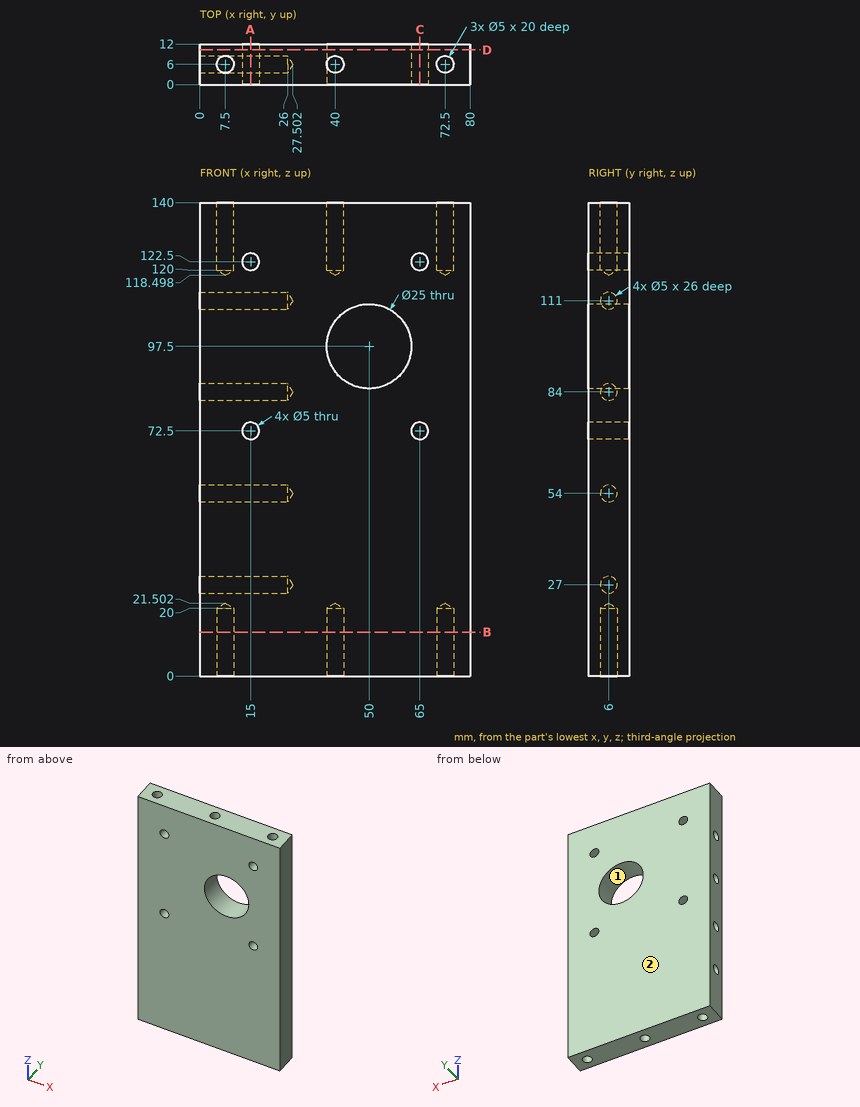
Here's the drawing with two shaded views (mm, measured from the low corner). I have some questions. Give positions to 0.01 mm unless a question says otherwise; leave off trailing zeros. Loops run counter-clockwise (first coordinate to the right, second up) from the corner with the lowest first, then second, coordinate; pieces in that order, holes last. Notation, with made-up numbers: (4, 20) - (52, 20) arc R35 cw to (52, 53) - close; hole circle Ø8 at (82, 28.5). An arc over 180 degrees is marked (long way). Return JSON: item names as keys, results as strings.
1. If I drill on line 1 (Z direction, x = 15, y = 3.25); line 2 (X direction, y = 6, z = 127); line 3 (Z direction, x = 18.75, y = 6), over which ranges is the centre line in solid material (lowest first)?
Output values:
{"line 1": "z = 0 to 70, 75 to 120, 125 to 140", "line 2": "x = 0 to 5, 10 to 37.5, 42.5 to 70, 75 to 80", "line 3": "z = 0 to 24.5, 29.5 to 51.5, 56.5 to 81.5, 86.5 to 108.5, 113.5 to 140"}
2. I want a section at D-D on y = 10.25. Please give me the cut outline in (x, z).
Output values:
{"outline": "(0, 0) - (80, 0) - (80, 140) - (0, 140) - close; hole circle Ø5 at (15, 72.5); hole circle Ø5 at (15, 122.5); hole circle Ø25 at (50, 97.5); hole circle Ø5 at (65, 72.5); hole circle Ø5 at (65, 122.5)"}
3. I want a section at C-C on x = 65. Please give me the cut outline in (y, z).
Output values:
{"outline": "(0, 0) - (12, 0) - (12, 70) - (0, 70) - close; (0, 75) - (12, 75) - (12, 120) - (0, 120) - close; (0, 125) - (12, 125) - (12, 140) - (0, 140) - close"}
4. I want a section at A-A on x = 15. Please give me the cut outline in (y, z).
Output values:
{"outline": "(0, 0) - (12, 0) - (12, 70) - (0, 70) - close; (0, 75) - (12, 75) - (12, 120) - (0, 120) - close; (0, 125) - (12, 125) - (12, 140) - (0, 140) - close; hole circle Ø5 at (6, 27); hole circle Ø5 at (6, 54); hole circle Ø5 at (6, 84); hole circle Ø5 at (6, 111)"}
5. We'd pull the mould along X, two halves only. Please class the marked faces 1 and 2: +X half, -X half, draft (parallel to the pull), parting line (faces both ways), or undercut.
Output values:
{"face 1": "undercut", "face 2": "draft"}
6. I want a section at B-B on z = 13. Please give me the cut outline in (x, y).
Output values:
{"outline": "(0, 0) - (80, 0) - (80, 12) - (0, 12) - close; hole circle Ø5 at (7.5, 6); hole circle Ø5 at (40, 6); hole circle Ø5 at (72.5, 6)"}
7. I'm going to push flat-ended pins straight in: pin 1 Ø3 at (x, y) = (40, 6) entering from +Z; pin 2 Ø4.5 at (x, y) = (7.5, 6) entering from -Z; pin 3 Ø15 at (x, z) = (50, 97.5) entering from +Y; pin 4 Ø4.5 at (y, z) = (6, 111) entering from -X. Where does each tip first touch, or does it pass through?
Output values:
{"pin 1": "stops at z = 119.4", "pin 2": "stops at z = 20.15", "pin 3": "passes through", "pin 4": "stops at x = 26.15"}
